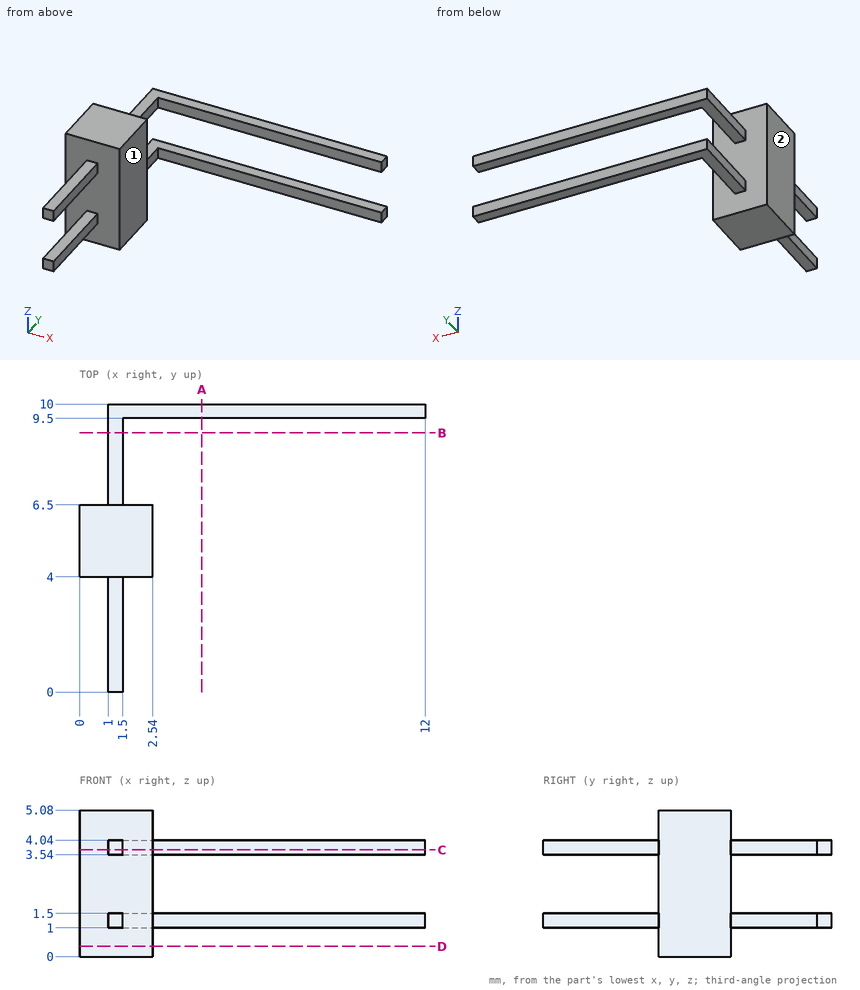
Geometry check sheet. Reference: drawing and pictorial views, mm from the part's lowest x, y, z. A direction names the side the tool comes from. Coordinates: 2 decimals unless noted, no trailing zeros. Order: outer loops, then holes, each group sorted by start corner. A loop starts at its lowest first (then second) coordinate and runs counter-clockwise, first axis right, second up. Notation, with made-up numbers: (77, 70.25) -> (128, 70.25) arc R19 cw to (128, 78.25) -> close; hole circle Ø11 at (16, 12.5). An arc over 180 degrees is marked (long way). Put each result on its own line as item: value. Start each with the question number.
1) Tool access check on the marked faces 1 and 2. Record the directions out of +Z, -Z, +X, -X, +Y, -Y that give a thin tool (end or side, any length) a straight path to the whole face; none if there is none.
2) Cross-section at C-C (z = 3.7). Enter the section's corners in (x, y), plus the area to 4 significant figures.
3) Cross-section at B-B (y = 9). Enter the section's corners in (x, z).
4) Material ranges on L1, parallel to Y at x = 1.25, z = 4.5; L2, parallel to X at y = 0.5, z = 1.05; L3, parallel to Y at x = 5.5, z = 1.05, recorded low to high.
5) Cross-section at D-D (z = 0.35). Enter the section's corners in (x, y).
6) Cross-section at A-A (x = 4.25). Enter the section's corners in (y, z).
7) Go/stop test with flat-tipped pins: pin 1 (1.5 mm diameter, centred on y = 7, z = 0.5, fed in from -X); pin 2 (0.6 mm diameter, centred on x = 1.5, y = 2, fed in from -Z); pin 3 (0.6 mm diameter, centred on y = 1.5, z = 1.5, fed in from +X); pin 4 (2 mm diameter, centred on y = 4.5, z = 2.5, fed in from +X). Record where each tip stops, or that it passes through.
Geometry check:
1. face 1: +Z, -Z, +X, -Y
1. face 2: +Z, -Z, -X, +Y, -Y
2. outline: (0, 4) -> (1, 4) -> (1, 0) -> (1.5, 0) -> (1.5, 4) -> (2.54, 4) -> (2.54, 6.5) -> (1.5, 6.5) -> (1.5, 9.5) -> (12, 9.5) -> (12, 10) -> (1, 10) -> (1, 6.5) -> (0, 6.5) -> close
2. area: 15.35 mm^2
3. outline: (1, 1) -> (1.5, 1) -> (1.5, 1.5) -> (1, 1.5) -> close; (1, 3.54) -> (1.5, 3.54) -> (1.5, 4.04) -> (1, 4.04) -> close
4. L1: y = 4 to 6.5
4. L2: x = 1 to 1.5
4. L3: y = 9.5 to 10
5. outline: (0, 4) -> (2.54, 4) -> (2.54, 6.5) -> (0, 6.5) -> close
6. outline: (9.5, 1) -> (10, 1) -> (10, 1.5) -> (9.5, 1.5) -> close; (9.5, 3.54) -> (10, 3.54) -> (10, 4.04) -> (9.5, 4.04) -> close
7. pin 1: stops at x = 0
7. pin 2: stops at z = 1
7. pin 3: stops at x = 1.5
7. pin 4: stops at x = 2.54
